Source: three-view drawing plus pictorial views. Frame: mm from the lowest corner of the part. A direction names the side the tool comes from. Give positions to 0.01 mm unless a question says otherwise; leave off trailing zeros. Write each loop counter-clockwise with the first axis right and the second up, starting at its lowest first coordinate (ties: lowest second). Pieces come first, ordered by that corner, then holes. Notation, with made-up numbers: (55, 47.25) -> (68, 47.25) arc R11 ccw to (68, 57.25) -> close; hole circle Ø5 at (-31.5, -19.75). An arc over 180 degrees is marked (long way). Answer in a Markdown table with one row per item. Add a question column.
Item 1: Material intervals for probe 1 along Y at (x, z) = (2.3, 3.2); probe 2 along Y at (x, z) = (2.1, 0.4); probe 3 along Z at (x, y) = (2.75, 12), sorted ascending. Write a range as from..to.
Item 2: First-contact query: P1, Ø2, axis at x = 2.5, y = 59, coming from the +Z side. Flat tip, straight axial feed; report the tip coordinate or a pass-through.
Item 3: Section query B-B on y = 7. Output: boundary loops of the cut face in (x, z).
Item 4: Section query A-A on z = 2.8. Output: boundary loops of the cut face in (x, y).
Item 5: Access query for the marked faces 1 and 2. Directions: +Z, -Z, +X, -X, +Y, -Y. A direction counts if a zero-diameter tool reaches every point of the face in a straight line with its end or side. Return the directions, or none.
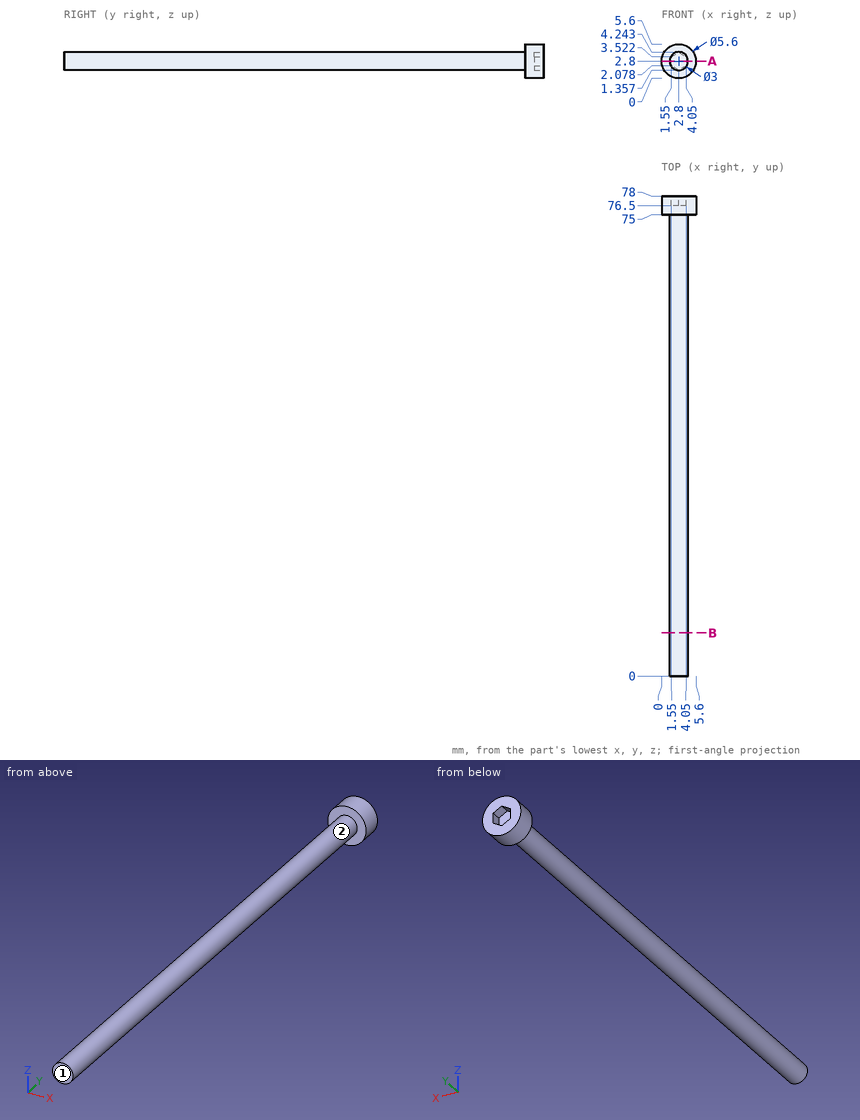
Findings below:
| question | item | result |
|---|---|---|
| 1 | probe 1 | y = 0..76.5 |
| 1 | probe 2 | y = 75..78 |
| 1 | probe 3 | z = 1.3..4.3 |
| 2 | P1 | stops at z = 4.3 |
| 3 | outline | circle Ø3 at (2.8, 2.8) |
| 4 | outline | (0, 75) -> (1.3, 75) -> (1.3, 0) -> (4.3, 0) -> (4.3, 75) -> (5.6, 75) -> (5.6, 78) -> (4.05, 78) -> (4.05, 76.5) -> (1.55, 76.5) -> (1.55, 78) -> (0, 78) -> close |
| 5 | face 1 | +Z, -Z, +X, -X, -Y |
| 5 | face 2 | -Y |
